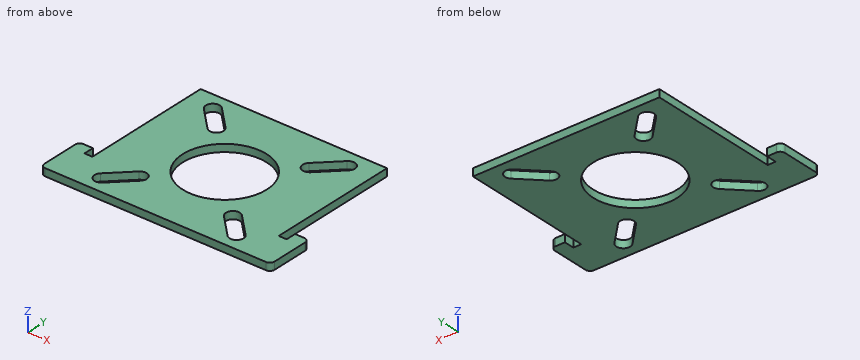
```python
from build123d import *

# Parameters (mm, degrees)
SKETCH1_W           = 40
SKETCH1_H           = 36
BOSS_EXTRUDE1_DEPTH = 1.6
LENSE_HOLE_R        = 9
CUT_EXTRUDE1_DEPTH  = 27.954776942
CUT_EXTRUDE2_DEPTH  = 27.954776942
BOSS_EXTRUDE2_DEPTH = 1.6
FILLET1_R           = 1


with BuildPart() as part:
    # Sketch1 → Boss-Extrude1 (new body)
    with BuildSketch(Plane.XY):
        Rectangle(SKETCH1_W, SKETCH1_H)
    extrude(amount=BOSS_EXTRUDE1_DEPTH)

    # lense hole → Cut-Extrude1 (cut, through all)
    with BuildSketch(Plane.XY):
        Circle(LENSE_HOLE_R)
    extrude(amount=CUT_EXTRUDE1_DEPTH, mode=Mode.SUBTRACT)

    # Sketch4 → Cut-Extrude2 (cut, through all)
    with BuildSketch(Plane.XY):
        with BuildLine():
            Line((-13.439339828, 15.560660172), (-8.939339828, 11.060660172))
            ThreePointArc((-8.939339828, 11.060660172), (-8.939339828, 8.939339828), (-11.060660172, 8.939339828))
            Line((-11.060660172, 8.939339828), (-15.560660172, 13.439339828))
            ThreePointArc((-15.560660172, 13.439339828), (-15.560660172, 15.560660172), (-13.439339828, 15.560660172))
        make_face()
        with BuildLine():
            Line((8.939339828, 11.060660172), (13.439339828, 15.560660172))
            ThreePointArc((13.439339828, 15.560660172), (15.560660172, 15.560660172), (15.560660172, 13.439339828))
            Line((15.560660172, 13.439339828), (11.060660172, 8.939339828))
            ThreePointArc((11.060660172, 8.939339828), (8.939339828, 8.939339828), (8.939339828, 11.060660172))
        make_face()
        with BuildLine():
            Line((11.060660172, -8.939339828), (15.560660172, -13.439339828))
            ThreePointArc((15.560660172, -13.439339828), (15.560660172, -15.560660172), (13.439339828, -15.560660172))
            Line((13.439339828, -15.560660172), (8.939339828, -11.060660172))
            ThreePointArc((8.939339828, -11.060660172), (8.939339828, -8.939339828), (11.060660172, -8.939339828))
        make_face()
        with BuildLine():
            Line((-15.560660172, -13.439339828), (-11.060660172, -8.939339828))
            ThreePointArc((-11.060660172, -8.939339828), (-8.939339828, -8.939339828), (-8.939339828, -11.060660172))
            Line((-8.939339828, -11.060660172), (-13.439339828, -15.560660172))
            ThreePointArc((-13.439339828, -15.560660172), (-15.560660172, -15.560660172), (-15.560660172, -13.439339828))
        make_face()
    extrude(amount=CUT_EXTRUDE2_DEPTH, mode=Mode.SUBTRACT)

    # Sketch5 → Boss-Extrude2 (add)
    with BuildSketch(Plane.XY):
        Polygon((20, -18), (24.7, -18), (24.7, -8), (21.7, -8), (21.7, -10.2), (20, -10.2), align=None)
    boss_extrude2 = extrude(amount=BOSS_EXTRUDE2_DEPTH)

    # Mirror1: Boss-Extrude2 across plane
    add(boss_extrude2.mirror(Plane(origin=(0, 0, 0), x_dir=(0, 0, 1), z_dir=(1, 0, 0))))

    # Fillet1
    fillet1_edges = [part.edges().sort_by_distance(p)[0] for p in [
        (24.7, -18, 0.8),
        (24.7, -8, 0.8),
        (-24.7, -18, 0.8),
        (-24.7, -8, 0.8),
    ]]
    fillet(fillet1_edges, radius=FILLET1_R)


solid = part.part
```
Check sheet for the modelled part. Datum: model origin and axes. Units: mm. Round coordinates to 2 decimals unless told otherwise and drop trailing zeros. Loops run counter-clockwise (first coordinate to the right, second up) from the corner with the lowest first, then second, coordinate; pieces in that order, holes last. Notation, with made-up numbers: (42, 15.25) - (48, 15.25) arc R25 cw to (48, 42.25) - close; hole circle Ø5 at (17, -36). An arc over 180 degrees is marked (long way). Write item = value, one per line. Start each with the question number.
Q1. Section check D-D (x = -14.5). Record the boundary of the cut face in (y, z), plus the area to 3 significant figures.
Q2. Section check A-A (y = 14.5). Record the boundary of the cut face in (x, z).
Q3. Thickness scan on L1, parallel to X at y = 0, z = 0.4; L2, parallel to Y at x = 0, z = 0.55; L3, parallel to X at y = 11.5, z = 0.25. Record the ranges inside material, lowest first.
Q4. Section check C-C (z = 1.15). Count the separate pieces of the cut face and the enclosed holes in it, plus the area to 3 significant figures.
Q5. Section check B-B (x = 0). Record the boundary of the cut face in (y, z).
Q6. Depth check by flat-ended pin: P1, Ø0.8, axis at x = 22.5, z = 1, coming from the +Y side; P2, Ø0.5, axis at y = 1, z = 1, coming from the -X side; P3, Ø0.5, axis at x = 20.5, z = 1, coming from the +Y side. Enter the tip coordinate at first touch or a pass-through.
Derived:
q1.outline = (-18, 0) - (-16, 0) - (-16, 1.6) - (-18, 1.6) - close; (-12.38, 0) - (12.38, 0) - (12.38, 1.6) - (-12.38, 1.6) - close; (16, 0) - (18, 0) - (18, 1.6) - (16, 1.6) - close
q1.area = 46.0 mm^2
q2.outline = (-20, 0) - (-16, 0) - (-16, 1.6) - (-20, 1.6) - close; (-12.38, 0) - (12.38, 0) - (12.38, 1.6) - (-12.38, 1.6) - close; (16, 0) - (20, 0) - (20, 1.6) - (16, 1.6) - close
q3.L1 = -20 to -9, 9 to 20
q3.L2 = -18 to -9, 9 to 18
q3.L3 = -20 to -13.62, -9.38 to 9.38, 13.62 to 20
q4.separate_pieces = 1
q4.enclosed_holes = 5
q4.area = 1,170 mm^2
q5.outline = (-18, 0) - (-9, 0) - (-9, 1.6) - (-18, 1.6) - close; (9, 0) - (18, 0) - (18, 1.6) - (9, 1.6) - close
q6.P1 = -8
q6.P2 = -20
q6.P3 = -10.2
